Geometry: final body of the model. Coordinates: model frame, mm. A direction names the side the tool comes from. Round coordinates to 2 decimals unless told otherwise and drop trailing zeros. Write each loop counter-clockwise with the first axis right and the second up, starting at its lowest first coordinate (ties: lowest second). Pieces come first, ordered by that corner, then holes. Notation, with made-up numbers: M 13.5,75.5 L 54.5,75.5 A13 cw 54.5,85.5 Z; hole C 28.25,34.5 d1. An arc over 180 degrees is marked long. Answer as CSV lines item,"result". Start each with the question number.
Q1. Section query D-D on y = -18. Output: boundary loops of the cut face in (x, z), and give its area (3 significant figures).
Q2. Mould query, pull axis X, two halves, no side actions, for faces 5 (the cylindrical face through (24.43, -22.53, 2.77)), 6 (the cylindrical face through (0.29, -6.77, 32.17)), 7 (the cylindrical face through (32.33, -19.35, 34.73)), 8 (the flat face through (9, -10, 0)). Classes: pulls with the +X half, pulls with the -X half, needs draft (parallel to the pull), parting line crosses it, or undercut.
Q3. Section query C-C on x = 6. Output: boundary loops of the cut face in (y, z).
Q4. Reachability of faces 1 (the flat face through (34, -14, 30.773)), 2 (the flat face through (24, -26, 8.796)), 3 (the flat face through (8, -9, 30.773)), 4 (the flat face through (22.365, -20, 20)) from +Z, -Z, +X, -X, +Y, -Y: full face, straight path, thin tool, end or side. Return the list, or none.
Q5. Section query B-B on z = 15. Output: boundary loops of the cut face in (x, y).
Q6. First-contact query: pin 1 (0.8 mm diameter, centred on x = 27.5, z = 32, fed in from -Y); pin 2 (3 mm diameter, centred on x = 25, z = 21.5, fed in from +Y); pin 3 (12 mm diameter, centred on y = -25.5, z = 15.5, fed in from -X). Flat tips, straight axial feed; report the tip coordinate or a pass-through.
Q7. Section query A-A on y = -25. Output: boundary loops of the cut face in (x, z).
Q8. Ray query, probe 1 along X at (y, z) = (-6.5, 34.5); probe 2 along Y at (x, z) = (25, 24); probe 3 along Z at (x, y) = (20.5, -6). Return the intervals inside material, ascending.
```python
from build123d import *

# Parameters (mm, degrees)
F0_W      = 38.1
F0_H      = 38.1
F1_DEPTH  = 38.1
F7_DEPTH  = 38.1
F8_DEPTH  = 38.1
F10_DEPTH = 38.1


with BuildPart() as f1:
    # F0 (on Front) → F1 (new body)
    with BuildSketch(Plane.XZ):
        with Locations((19.05, 19.05)):
            Rectangle(F0_W, F0_H)
    extrude(amount=F1_DEPTH)

    # F6 (on offset) → F7 (cut)
    with BuildSketch(Plane.YZ.offset(38.1)):
        with BuildLine():
            Line((-20.187413, 31.75), (-29.192599, 31.75))
            Line((-29.192599, 31.75), (-35.52093, 31.75))
            ThreePointArc((-35.52093, 31.75), (-37.267369, 32.473399), (-37.990768, 34.219837))
            Line((-37.990768, 34.219837), (-37.990768, 35.630163))
            ThreePointArc((-37.990768, 35.630163), (-37.267369, 37.376601), (-35.52093, 38.1))
            Line((-35.52093, 38.1), (-38.1, 38.1))
            Line((-38.1, 38.1), (-38.1, 15.848642))
            ThreePointArc((-38.1, 15.848642), (-37.376601, 17.595081), (-35.630163, 18.31848))
            Line((-35.630163, 18.31848), (-34.611057, 18.31848))
            ThreePointArc((-34.611057, 18.31848), (-32.883701, 17.613958), (-32.141803, 15.902322))
            Line((-32.141803, 15.902322), (-32.039838, 11.211913))
            ThreePointArc((-32.039838, 11.211913), (-31.29794, 9.500277), (-29.570584, 8.795755))
            Line((-29.570584, 8.795755), (-22.657251, 8.795755))
            ThreePointArc((-22.657251, 8.795755), (-20.910812, 9.519154), (-20.187413, 11.265592))
            Line((-20.187413, 11.265592), (-20.187413, 31.75))
        make_face()
        with BuildLine():
            Line((0, 0), (0, 34.219837))
            ThreePointArc((0, 34.219837), (-0.723399, 32.473399), (-2.469837, 31.75))
            Line((-2.469837, 31.75), (-7.248927, 31.75))
            Line((-7.248927, 31.75), (-7.248927, 2.469837))
            ThreePointArc((-7.248927, 2.469837), (-7.972326, 0.723399), (-9.718765, 0))
            Line((-9.718765, 0), (0, 0))
        make_face()
        with BuildLine():
            Line((0, 38.1), (-2.469837, 38.1))
            ThreePointArc((-2.469837, 38.1), (-0.723399, 37.376601), (0, 35.630163))
            Line((0, 35.630163), (0, 38.1))
        make_face()
        with BuildLine():
            ThreePointArc((-35.630163, 0), (-37.376601, 0.723399), (-38.1, 2.469837))
            Line((-38.1, 2.469837), (-38.1, 0))
            Line((-38.1, 0), (-35.630163, 0))
        make_face()
    extrude(amount=-F7_DEPTH, mode=Mode.SUBTRACT)

    # F5 (on offset) → F8 (cut)
    with BuildSketch(Plane.XZ.offset(38.1)):
        with BuildLine():
            Line((0, 38.1), (0, 13.888076))
            ThreePointArc((0, 13.888076), (0.723399, 15.634515), (2.469837, 16.357914))
            Line((2.469837, 16.357914), (3.4497, 16.357914))
            ThreePointArc((3.4497, 16.357914), (3.813439, 16.20421), (3.95674, 15.83625))
            ThreePointArc((3.95674, 15.83625), (5.750677, 11.229898), (10.304174, 9.30575))
            Line((10.304174, 9.30575), (11.1735, 9.30575))
            Line((11.1735, 9.30575), (12.626726, 9.30575))
            ThreePointArc((12.626726, 9.30575), (17.116854, 11.165622), (18.976726, 15.65575))
            Line((18.976726, 15.65575), (18.976726, 24.423077))
            ThreePointArc((18.976726, 24.423077), (17.116854, 28.913205), (12.626726, 30.773077))
            Line((12.626726, 30.773077), (12.052785, 30.773077))
            Line((12.052785, 30.773077), (2.512986, 30.773077))
            ThreePointArc((2.512986, 30.773077), (0.766547, 31.496476), (0.043148, 33.242915))
            Line((0.043148, 33.242915), (0.043148, 35.630163))
            ThreePointArc((0.043148, 35.630163), (0.766547, 37.376601), (2.512986, 38.1))
            Line((2.512986, 38.1), (0, 38.1))
        make_face()
        with BuildLine():
            ThreePointArc((25.53427, 6.35), (23.674398, 1.859872), (19.18427, 0))
            Line((19.18427, 0), (38.1, 0))
            Line((38.1, 0), (38.1, 38.1))
            Line((38.1, 38.1), (35.599574, 38.1))
            ThreePointArc((35.599574, 38.1), (37.337263, 37.385307), (38.069288, 35.654848))
            Line((38.069288, 35.654848), (38.093149, 33.2676))
            ThreePointArc((38.093149, 33.2676), (37.37858, 31.505225), (35.623435, 30.773077))
            Line((35.623435, 30.773077), (31.88427, 30.773077))
            ThreePointArc((31.88427, 30.773077), (27.394142, 28.913205), (25.53427, 24.423077))
            Line((25.53427, 24.423077), (25.53427, 6.35))
        make_face()
    extrude(amount=-F8_DEPTH, mode=Mode.SUBTRACT)

    # F9 (on offset) → F10 (cut)
    with BuildSketch(Plane.XY.offset(38.1)):
        with BuildLine():
            Line((27.78691, -17.437199), (26.787849, -17.437199))
            Line((26.787849, -17.437199), (26.787849, -32.756366))
            Line((26.787849, -32.756366), (27.78691, -32.756366))
            ThreePointArc((27.78691, -32.756366), (32.277038, -30.896494), (34.13691, -26.406366))
            Line((34.13691, -26.406366), (34.13691, -23.787199))
            ThreePointArc((34.13691, -23.787199), (32.277038, -19.297071), (27.78691, -17.437199))
        make_face()
        with BuildLine():
            Line((38.1, 0), (31.75, 0))
            ThreePointArc((31.75, 0), (36.240128, -1.859872), (38.1, -6.35))
            Line((38.1, -6.35), (38.1, 0))
        make_face()
        with BuildLine():
            Line((16.014762, -10.832123), (0, -10.832123))
            Line((0, -10.832123), (0, -38.23876))
            Line((0, -38.23876), (0.831124, -38.23876))
            Line((0.831124, -38.23876), (28.714762, -38.23876))
            ThreePointArc((28.714762, -38.23876), (24.224634, -36.378888), (22.364762, -31.88876))
            Line((22.364762, -31.88876), (22.364762, -31.69275))
            Line((22.364762, -31.69275), (22.364762, -17.182123))
            ThreePointArc((22.364762, -17.182123), (20.50489, -12.691995), (16.014762, -10.832123))
        make_face()
    extrude(amount=-F10_DEPTH, mode=Mode.SUBTRACT)


solid = f1.part
```
Entries:
1,outline,"M 22.36,0.85 A6.35 ccw 25.53,6.35 L 25.53,24.42 A6.35 cw 26.79,28.21 L 26.79,38.1 L 22.36,38.1 Z; M 30.4,30.6 A6.35 cw 31.88,30.77 L 35.62,30.77 A2.47 ccw 38.09,33.27 L 38.07,35.65 A2.47 ccw 35.6,38.1 L 30.4,38.1 Z"
1,area,"181 mm^2"
2,face 5,"pulls with the +X half"
2,face 6,"pulls with the -X half"
2,face 7,"undercut"
2,face 8,"needs draft"
3,outline,"M -10.83,0 L -9.72,0 A2.47 ccw -7.25,2.47 L -7.25,10.99 L -10.83,10.99 Z; M -10.83,30.77 L -7.25,30.77 L -7.25,31.75 L -2.47,31.75 A2.47 ccw 0,34.22 L 0,35.63 A2.47 ccw -2.47,38.1 L -10.83,38.1 Z"
4,face 1,"-Z, +X, +Y, -Y"
4,face 2,"+X, -X"
4,face 3,"-X, +Y, -Y"
4,face 4,"+Z, -Z, -X, -Y"
5,outline,"M 0.26,-10.83 L 3.99,-10.83 L 3.99,-7.25 L 0.26,-7.25 Z; M 18.94,-11.55 A6.35 cw 22.36,-17.18 L 22.36,-20.19 L 25.53,-20.19 L 25.53,-7.25 L 18.94,-7.25 Z; M 22.37,-32.12 A6.35 ccw 25.53,-37.38 L 25.53,-32.12 Z"
6,pin 1,"stops at y = -37.19"
6,pin 2,"stops at y = -7.25"
6,pin 3,"stops at x = 22.36"
7,outline,"M 22.36,0.85 A6.35 ccw 25.53,6.35 L 25.53,8.8 L 22.36,8.8 Z; M 22.36,31.75 L 26.79,31.75 L 26.79,38.1 L 22.36,38.1 Z; M 34.14,31.75 L 37.59,31.75 A2.47 ccw 38.09,33.27 L 38.07,35.65 A2.47 ccw 35.6,38.1 L 34.14,38.1 Z"
8,probe 1,"x = 0.04 to 38.08"
8,probe 2,"y = -20.19 to -7.25"
8,probe 3,"z = 31.75 to 38.1"
